The listing builds one solid part. Answer for the finished solid, in the listing's coordinates (mm). Face numbers are marked on the shaded views. A direction names the side the tool comes from. Coordinates: 2 decimals unless noted, no trailing zeros. Write each loop counter-clockwise with the first axis right and the second up, starting at its lowest first coordinate (ties: lowest second). Pieces come first, ordered by that corner, then holes.
from build123d import *

# Parameters (mm, degrees)
SKETCH2_R                = 33.8
CUT_EXTRUDE1_DEPTH       = 19.1
CUT_EXTRUDE2_START       = -33.8
CUT_EXTRUDE2_DEPTH       = 14.7
BOSS_EXTRUDE2_START      = -2.2
BOSS_EXTRUDE2_DEPTH      = 2.2
CUT_EXTRUDE3_REACH       = 42.08
SKETCH6_R                = 1.6
SKETCH19_R               = 9
CUT_EXTRUDE10_DEPTH      = 1.4
CUT_EXTRUDE11_REACH      = 42.429
CUT_EXTRUDE11_END_RADIUS = 33.8
SKETCH20_R               = 3.5
CUT_EXTRUDE9_REACH       = 44.024
CUT_EXTRUDE9_END_RADIUS  = 33.8
CUT_EXTRUDE7_REACH       = 44.024
CUT_EXTRUDE7_END_RADIUS  = 33.8
SKETCH10_R               = 1.45
SKETCH14_W               = 10
SKETCH14_H               = 1
BOSS_EXTRUDE1_DEPTH      = 3
CUT_EXTRUDE12_START      = -10.118299
SKETCH21_R               = 27.886018002
CUT_EXTRUDE12_DEPTH      = 10.118299


with BuildPart() as part:
    # Sketch1 → Revolve1 (revolve)
    with BuildSketch(Plane.XY, mode=Mode.PRIVATE) as revolve1_sk:
        with BuildLine():
            Line((0, -33.8), (0, 0))
            Line((0, 0), (33.8, 0))
            ThreePointArc((33.8, 0), (23.900209204, -23.900209204), (0, -33.8))
        make_face()
    revolve(revolve1_sk.sketch.rotate(Axis((0, -33.8, 0), (0, 1, 0)), 180), axis=Axis((0, -33.8, 0), (0, 1, 0)))

    # Sketch2 → Cut-Extrude1 (cut)
    with BuildSketch(Plane(origin=(0, 0, 0), x_dir=(1, 0, 0), z_dir=(0, 1, 0))):
        Circle(SKETCH2_R)
    extrude(amount=-CUT_EXTRUDE1_DEPTH, mode=Mode.SUBTRACT)

    # Sketch5 → Cut-Extrude2 (cut)
    with BuildSketch(Plane(origin=(0, 0, 0), x_dir=(1, 0, 0), z_dir=(0, 1, 0)).offset(CUT_EXTRUDE2_START)):
        with BuildLine():
            Line((-17.025732229, 6.571677263), (-23.544283672, 3.742739979))
            ThreePointArc((-23.544283672, 3.742739979), (-23.775794442, 3.633514413), (-24, 3.509985755))
            Line((-24, 3.509985755), (-24, -3.509985755))
            ThreePointArc((-24, -3.509985755), (-23.775794442, -3.633514413), (-23.544283672, -3.742739979))
            Line((-23.544283672, -3.742739979), (-17.025732229, -6.571677263))
            ThreePointArc((-17.025732229, -6.571677263), (0, -18.25), (17.025732229, -6.571677263))
            Line((17.025732229, -6.571677263), (23.544283672, -3.742739979))
            ThreePointArc((23.544283672, -3.742739979), (23.775794442, -3.633514413), (24, -3.509985755))
            Line((24, -3.509985755), (24, 3.509985755))
            ThreePointArc((24, 3.509985755), (23.775794442, 3.633514413), (23.544283672, 3.742739979))
            Line((23.544283672, 3.742739979), (17.025732229, 6.571677263))
            ThreePointArc((17.025732229, 6.571677263), (0, 18.25), (-17.025732229, 6.571677263))
        make_face()
    extrude(amount=CUT_EXTRUDE2_DEPTH, mode=Mode.SUBTRACT)

    # Sketch16 → Boss-Extrude2 (add)
    with BuildSketch(Plane(origin=(0, -19.1, 0), x_dir=(1, 0, 0), z_dir=(0, 1, 0)).offset(BOSS_EXTRUDE2_START)):
        with BuildLine():
            Line((17.025732229, 6.571677263), (23.544283672, 3.742739979))
            ThreePointArc((23.544283672, 3.742739979), (23.775794442, 3.633514413), (24, 3.509985755))
            Line((24, 3.509985755), (24, -3.509985755))
            ThreePointArc((24, -3.509985755), (23.775794442, -3.633514413), (23.544283672, -3.742739979))
            Line((23.544283672, -3.742739979), (17.025732229, -6.571677263))
            ThreePointArc((17.025732229, -6.571677263), (18.25, 0), (17.025732229, 6.571677263))
        make_face()
        with BuildLine():
            Line((-23.544283672, -3.742739979), (-17.025732229, -6.571677263))
            ThreePointArc((-17.025732229, -6.571677263), (-18.25, 0), (-17.025732229, 6.571677263))
            Line((-17.025732229, 6.571677263), (-23.544283672, 3.742739979))
            ThreePointArc((-23.544283672, 3.742739979), (-23.775794442, 3.633514413), (-24, 3.509985755))
            Line((-24, 3.509985755), (-24, -3.509985755))
            ThreePointArc((-24, -3.509985755), (-23.775794442, -3.633514413), (-23.544283672, -3.742739979))
        make_face()
    extrude(amount=BOSS_EXTRUDE2_DEPTH)

    # Sketch6 → Cut-Extrude3 (cut, up to next)
    with BuildSketch(Plane(origin=(0, -21.3, 0), x_dir=(1, 0, 0), z_dir=(0, 1, 0)), mode=Mode.PRIVATE) as cut_extrude3_sk1:
        with Locations(Location((-21.92, 0, 0), (0, 0, 270))):
            Circle(SKETCH6_R)
    cut_extrude3_tool1 = extrude(cut_extrude3_sk1.sketch, amount=CUT_EXTRUDE3_REACH, mode=Mode.PRIVATE) & part.part
    # Sketch6 → Cut-Extrude3 (cut, up to next)
    with BuildSketch(Plane(origin=(0, -21.3, 0), x_dir=(1, 0, 0), z_dir=(0, 1, 0)), mode=Mode.PRIVATE) as cut_extrude3_sk2:
        with Locations(Location((21.92, 0, 0), (0, 0, 270))):
            Circle(SKETCH6_R)
    cut_extrude3_tool2 = extrude(cut_extrude3_sk2.sketch, amount=CUT_EXTRUDE3_REACH, mode=Mode.PRIVATE) & part.part
    add(cut_extrude3_tool1.solids().sort_by_distance((-21.92, -21.3, 0))[0], mode=Mode.SUBTRACT)
    add(cut_extrude3_tool2.solids().sort_by_distance((21.92, -21.3, 0))[0], mode=Mode.SUBTRACT)

    # Revolve2: read off the stored shape, not the designer's step
    # Revolve2 outline → Revolve2 (revolve)
    with BuildSketch(Plane.XY):
        with BuildLine():
            Line((0, -23.5), (0, -33.8))
            ThreePointArc((0, -33.8), (13.168073663, -31.129436808), (24.255308697, -23.53975361))
            Line((24.255308697, -23.53975361), (24.255308697, -23.5))
            Line((24.255308697, -23.5), (0, -23.5))
        make_face()
    revolve(axis=Axis((0, 0, 0), (0, 1, 0)))

    # Sketch19 → Cut-Extrude10 (cut)
    with BuildSketch(Plane(origin=(0, -23.5, 0), x_dir=(1, 0, 0), z_dir=(0, 1, 0))):
        with Locations(Location((0, 0, 0), (0, 0, 180))):
            Circle(SKETCH19_R)
    extrude(amount=-CUT_EXTRUDE10_DEPTH, mode=Mode.SUBTRACT)

    # Cut-Extrude11: up to this sphere (the profile starts inside it)
    cut_extrude11_end = Location((0, 0, 0)) * Sphere(CUT_EXTRUDE11_END_RADIUS, mode=Mode.PRIVATE)
    # Sketch20 → Cut-Extrude11 (cut, up to the surface)
    with BuildSketch(Plane(origin=(0, -24.9, 0), x_dir=(1, 0, 0), z_dir=(0, 1, 0)), mode=Mode.PRIVATE) as cut_extrude11_sk1:
        with Locations(Location((0, 0, 0), (0, 0, 180))):
            Circle(SKETCH20_R)
    cut_extrude11_tool1 = extrude(cut_extrude11_sk1.sketch, amount=-CUT_EXTRUDE11_REACH, mode=Mode.PRIVATE) & cut_extrude11_end
    add(cut_extrude11_tool1.solids().sort_by_distance((0, -24.9, 0))[0], mode=Mode.SUBTRACT)

    # Cut-Extrude9: up to this sphere (the profile starts inside it)
    cut_extrude9_end = Location((0, 0, 0)) * Sphere(CUT_EXTRUDE9_END_RADIUS, mode=Mode.PRIVATE)
    # Sketch13 → Cut-Extrude9 (cut, up to the surface)
    with BuildSketch(Plane(origin=(0, -19.1, 0), x_dir=(1, 0, 0), z_dir=(0, 1, 0)), mode=Mode.PRIVATE) as cut_extrude9_sk1:
        Polygon((10.556374993, -19.224020053), (13.210464636, -21.224020053), (17.724077309, -15.234253728), (16.925441799, -14.632438705), (18.730886869, -12.236532175), (19.529522379, -12.838347198), (24.043135053, -6.848580873), (21.389045409, -4.848580873), align=None)
    cut_extrude9_tool1 = extrude(cut_extrude9_sk1.sketch, amount=-CUT_EXTRUDE9_REACH, mode=Mode.PRIVATE) & cut_extrude9_end
    add(cut_extrude9_tool1.solids().sort_by_distance((17.250772, -19.1, 12.999389))[0], mode=Mode.SUBTRACT)

    # Cut-Extrude7: up to this sphere (the profile starts inside it)
    cut_extrude7_end = Location((0, 0, 0)) * Sphere(CUT_EXTRUDE7_END_RADIUS, mode=Mode.PRIVATE)
    # Sketch10 → Cut-Extrude7 (cut, up to the surface)
    with BuildSketch(Plane(origin=(0, -19.1, 0), x_dir=(1, 0, 0), z_dir=(0, 1, 0)), mode=Mode.PRIVATE) as cut_extrude7_sk1:
        with Locations(Location((-23.49231552, -8.550503583, 0), (0, 0, 270))):
            Circle(SKETCH10_R)
    cut_extrude7_tool1 = extrude(cut_extrude7_sk1.sketch, amount=-CUT_EXTRUDE7_REACH, mode=Mode.PRIVATE) & cut_extrude7_end
    add(cut_extrude7_tool1.solids().sort_by_distance((-23.492316, -19.1, 8.550504))[0], mode=Mode.SUBTRACT)
    # Sketch10 → Cut-Extrude7 (cut, up to the surface)
    with BuildSketch(Plane(origin=(0, -19.1, 0), x_dir=(1, 0, 0), z_dir=(0, 1, 0)), mode=Mode.PRIVATE) as cut_extrude7_sk2:
        with Locations(Location((23.49231552, 8.550503583, 0), (0, 0, 270))):
            Circle(SKETCH10_R)
    cut_extrude7_tool2 = extrude(cut_extrude7_sk2.sketch, amount=-CUT_EXTRUDE7_REACH, mode=Mode.PRIVATE) & cut_extrude7_end
    add(cut_extrude7_tool2.solids().sort_by_distance((23.492316, -19.1, -8.550504))[0], mode=Mode.SUBTRACT)

    # Sketch14 → Boss-Extrude1 (add)
    with BuildSketch(Plane(origin=(0, -19.1, 0), x_dir=(1, 0, 0), z_dir=(0, 1, 0))):
        with Locations((12, 17.911516357)):
            Rectangle(SKETCH14_W, SKETCH14_H)
        with Locations((-11, 17.911516357)):
            Rectangle(SKETCH14_W, SKETCH14_H)
    extrude(amount=BOSS_EXTRUDE1_DEPTH)

    # Sketch21 → Cut-Extrude12 (cut)
    with BuildSketch(Plane(origin=(0, -23.5, 0), x_dir=(1, 0, 0), z_dir=(0, 1, 0)).offset(CUT_EXTRUDE12_START)):
        Circle(SKETCH21_R)
    extrude(amount=CUT_EXTRUDE12_DEPTH, mode=Mode.SUBTRACT)


solid = part.part
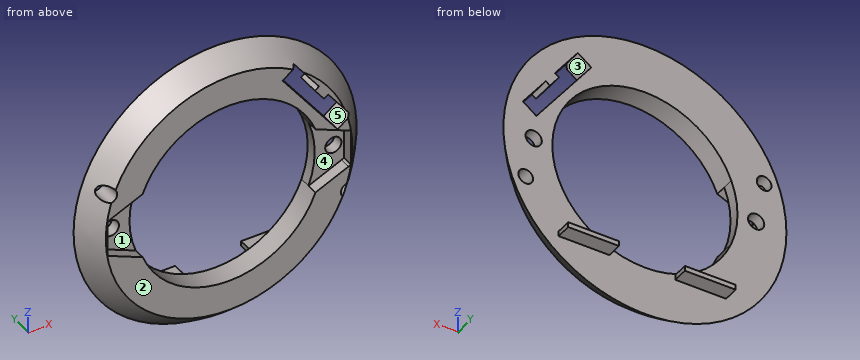
Q1. The part is cut by section B-B, the plane x = -14. Write down the section's boundary in (y, z), then the cut area to 3 significant figures.
Answers below:
outline: (-23.5, -19.85) arc R30.76 ccw to (-19.1, -24.12) - (-19.1, -18.41) - (-16.1, -18.41) - (-16.1, -17.41) - (-19.1, -17.41) - (-19.1, -11.71) - (-23.5, -11.71) - close; (-23.5, 11.71) - (-19.1, 11.71) - (-19.1, 24.12) arc R30.76 ccw to (-23.5, 19.85) - close
area: 94.7 mm2
Q2. The part is cut by section C-C, the plane y = -18. Write down the section's boundary in (x, z), then the cut area to 3 significant figures.
Answers below:
outline: (-16, -18.41) - (-6, -18.41) - (-6, -17.41) - (-16, -17.41) - close; (7, -18.41) - (17, -18.41) - (17, -17.41) - (7, -17.41) - close
area: 20.0 mm2
Q3. The part is cut by section D-D, the plane z = 16.5. Write down the section's boundary in (x, y), then the cut area to 3 significant figures.
Answers below:
outline: (-22.48, -19.1) arc R29.5 ccw to (-17.83, -23.5) - (-7.8, -23.5) - (-7.8, -19.1) - close; (7.8, -23.5) - (12.61, -23.5) - (12.61, -19.1) - (7.8, -19.1) - close; (16.77, -23.5) - (17.83, -23.5) arc R29.5 ccw to (22.48, -19.1) - (16.77, -19.1) - close
area: 91.9 mm2
Q4. Which of the six approach directions +Z, -Z, +X, -X, +Y, -Y give full straight-line access (tool end or side, diameter ignored) to the marked faces 4 and 5?
Answers below:
face 4: -Y
face 5: +Y, -Y
Q5. The part is cut by section A-A, the plane z = 0. Write down the section's boundary in (x, y).
Answers below:
outline: (-27.89, -19.1) arc R33.8 ccw to (-24.29, -23.5) - (-24, -23.5) - (-24, -21.3) - (-23.52, -21.3) - (-23.52, -19.1) - close; (-20.32, -21.3) - (-18.25, -21.3) - (-18.25, -19.1) - (-20.32, -19.1) - close; (18.25, -21.3) - (20.32, -21.3) - (20.32, -19.1) - (18.25, -19.1) - close; (23.52, -21.3) - (24, -21.3) - (24, -23.5) - (24.29, -23.5) arc R33.8 ccw to (27.89, -19.1) - (23.52, -19.1) - close
Q6. Determine the mould class of the marked faces 1, 2 and 3 for opening direction X: released by +X, released by -X, zero draft, split by the parting line, or undercut.
Answers below:
face 1: undercut
face 2: zero draft
face 3: undercut
Q7. Given pin 1 (8 mm diameter, centred on x = -14.5, z = -7, fed in from +Y); pin 2 (2.5 mm diameter, centred on x = 13, y = -17.5, fed in from +Z); pin 3 (3 mm diameter, centred on x = 21.92, z = 0, fed in from -Y); pin 4 (1 mm diameter, centred on y = -22, z = 5, fed in from -X), each flat-ended and moving along its own axis, determine where each tip first touches the part or whether it passes through.
Answers below:
pin 1: stops at y = -19.1
pin 2: stops at z = -17.41
pin 3: passes through
pin 4: stops at x = -25.61
Q8. Find the intervals of material crossed by probe 1 along Z at (x, y) = (21.92, -19.85); probe 2 along Z at (x, y) = (21.5, -22.25); probe 3 along Y at (x, z) = (21.5, 4.5), in increasing order.
Answers below:
probe 1: z = -16.37 to -1.6, 1.6 to 5.25, 9.67 to 16.37
probe 2: z = -13.61 to -4.63, 4.63 to 4.93, 10.22 to 13.61
probe 3: y = -21.3 to -19.1
